from build123d import *

# Parameters (mm, degrees)
SKETCH001_W   = 0.48
SKETCH001_H   = 0.38
PAD001_DEPTH  = 5
PAD_DEPTH     = 4.8
SKETCH002_W   = 0.48
SKETCH002_H   = 4.3
SKETCH002_H_2 = 5.57
PAD002_DEPTH  = 0.38
FILLET_R      = 0.35


with BuildPart() as pad001:
    # Sketch001 → Pad001 (new body)
    with BuildSketch(Plane.XY.offset(1.4)):
        Rectangle(SKETCH001_W, SKETCH001_H)
        with Locations((1.27, 1.27)):
            Rectangle(SKETCH001_W, SKETCH001_H)
        with Locations((2.54, 0)):
            Rectangle(SKETCH001_W, SKETCH001_H)
    extrude(amount=-PAD001_DEPTH)


with BuildPart() as pad:
    # Sketch → Pad (new body)
    with BuildSketch(Plane(origin=(0, -4, 1.4), x_dir=(1, 0, 0), z_dir=(0, -1, 0))):
        with BuildLine():
            Line((-0.745769, -1.33), (3.285769, -1.33))
            ThreePointArc((3.285769, -1.33), (1.27, 2.415), (-0.745769, -1.33))
        make_face()
    extrude(amount=PAD_DEPTH)


with BuildPart() as obj1:
    # Sketch002 → Pad002 (new body)
    with BuildSketch(Plane.XY.offset(1.4)):
        with Locations((2.54, -1.96)):
            Rectangle(SKETCH002_W, SKETCH002_H)
        with Locations((1.27, -1.325)):
            Rectangle(SKETCH002_W, SKETCH002_H_2)
        with Locations((0, -1.96)):
            Rectangle(SKETCH002_W, SKETCH002_H)
    extrude(amount=PAD002_DEPTH)

    # Fillet
    fillet_edges = [obj1.edges().sort_by_distance(p)[0] for p in [
        (2.54, 0.19, 1.78),
        (0, 0.19, 1.78),
        (1.27, 1.46, 1.78),
    ]]
    fillet(fillet_edges, radius=FILLET_R)

    # obj1: union Pad001, Pad
    add(pad001.part)
    add(pad.part)


solid = obj1.part
Verification items for the finished model (mm, model axes). A direction names the side the tool comes from. Coordinates: 2 decimals unless noted, no trailing zeros. Write each loop counter-clockwise with the first axis right and the second up, starting at its lowest first coordinate (ties: lowest second). Pieces come first, ordered by that corner, then holes. Notation, with made-up numbers: (39, 43.25) -> (91, 43.25) arc R17 ccw to (91, 58.25) -> close; hole circle Ø7 at (60, 42.5). An arc over 180 degrees is marked (long way). One line per item, written item: value. Start each with the question number.
Q1. Cross-section at C-C on z = 1.25. Enter the section's corners in (x, y).
Q2. Cross-section at B-B on z = -0.25. Enter the section's corners in (x, y), and give its area (3 significant figures).
Q3. Mould release check, pull along Y, two halves, no side actions. Record for faces 5 (the flat face through (1, -8.8, 2)), 6 (the flat face through (2.78, 0, 0)), 7 (the flat face through (1, -4, 2)): pulls with the +Y half, pulls with the -Y half, needs draft (parallel to the pull), parting line crosses it, or undercut.
Q4. Thickness scan on L1, parallel to X at y = -0.5, z = 1.5; L2, parallel to Y at x = 2.35, z = -2.5; L3, parallel to Y at x = 3.25, z = 1. Record the ranges inside material, lowest first. Write a range as from..to.
Q5. Cross-section at A-A on y = -3. Enter the section's corners in (x, z), and give its area (3 significant figures).
Q6. Go/stop test with flat-tipped pins: P1, Ø3.5, axis at y = -3, z = -0.5, coming from the -X side; P2, Ø1.5, axis at y = 0, z = -3, coming from the +X side; P3, Ø2.5, axis at y = -0.5, z = -1.5, coming from the -X side. Record where each tip stops, or that it passes through.
Q7. Access from +Z, -Z, +X, -X, +Y, -Y to the whole of each face (thin tool, end or side, straight path). Record for faces 1 (the flat face through (0.24, 0, 0)), 2 (the cylindrical face through (1.343, -6.366, 3.814)), 3 (the flat face through (1, -6, 0.07)), 4 (the flat face through (-0.24, 0, 0)).
Q8. Cross-section at D-D on x = 1.27. Enter the section's corners in (y, z) (3 decimals), and give its area (3 significant figures).
Checked values:
1. outline: (-1.14, -8.8) -> (3.68, -8.8) -> (3.68, -4) -> (-1.14, -4) -> close; (-0.24, -0.19) -> (0.24, -0.19) -> (0.24, 0.19) -> (-0.24, 0.19) -> close; (1.03, 1.08) -> (1.51, 1.08) -> (1.51, 1.46) -> (1.03, 1.46) -> close; (2.3, -0.19) -> (2.78, -0.19) -> (2.78, 0.19) -> (2.3, 0.19) -> close
2. outline: (-0.24, -0.19) -> (0.24, -0.19) -> (0.24, 0.19) -> (-0.24, 0.19) -> close; (1.03, 1.08) -> (1.51, 1.08) -> (1.51, 1.46) -> (1.03, 1.46) -> close; (2.3, -0.19) -> (2.78, -0.19) -> (2.78, 0.19) -> (2.3, 0.19) -> close
2. area: 0.547 mm²
3. face 5: pulls with the -Y half
3. face 6: needs draft
3. face 7: undercut
4. L1: x = -0.24..0.24, 1.03..1.51, 2.3..2.78
4. L2: y = -0.19..0.19
4. L3: y = -8.8..-4
5. outline: (-0.24, 1.4) -> (0.24, 1.4) -> (0.24, 1.78) -> (-0.24, 1.78) -> close; (1.03, 1.4) -> (1.51, 1.4) -> (1.51, 1.78) -> (1.03, 1.78) -> close; (2.3, 1.4) -> (2.78, 1.4) -> (2.78, 1.78) -> (2.3, 1.78) -> close
5. area: 0.547 mm²
6. P1: stops at x = -1.1
6. P2: stops at x = 2.78
6. P3: stops at x = -0.24
7. face 1: +Z, -Z, +Y
7. face 2: +Y, -Y
7. face 3: -Z, +X, -X, -Y
7. face 4: +Z, -Z, -X, +Y
8. outline: (-8.8, 0.07) -> (-4, 0.07) -> (-4, 1.4) -> (1.08, 1.4) -> (1.08, -3.6) -> (1.46, -3.6) -> (1.46, 1.43) arc R0.35 ccw to (1.11, 1.78) -> (-4, 1.78) -> (-4, 3.815) -> (-8.8, 3.815) -> close
8. area: 21.9 mm²
